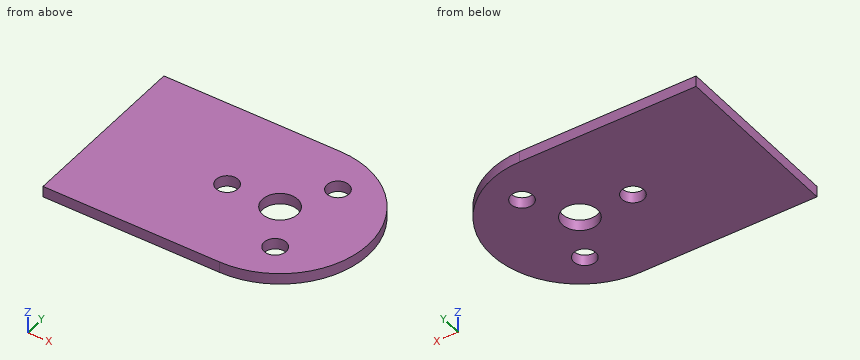
```python
from build123d import *

# Parameters (mm, degrees)
SKETCH1_R           = 5.08
SKETCH1_R_2         = 3.175
BOSS_EXTRUDE1_DEPTH = 3.175


with BuildPart() as part:
    # Sketch1 → Boss-Extrude1 (new body)
    with BuildSketch(Plane.XY):
        with BuildLine():
            Line((22.225, 50.613247917), (-28.575, 50.613247917))
            Line((-28.575, 50.613247917), (-28.575, 101.413247917))
            Line((-28.575, 101.413247917), (22.225, 101.413247917))
            ThreePointArc((22.225, 101.413247917), (47.625, 76.013247917), (22.225, 50.613247917))
        make_face()
        with Locations((22.225, 76.013247917)):
            Circle(SKETCH1_R, mode=Mode.SUBTRACT)
        with Locations((6.985, 76.013247917)):
            Circle(SKETCH1_R_2, mode=Mode.SUBTRACT)
        with Locations((29.845, 89.211475071)):
            Circle(SKETCH1_R_2, mode=Mode.SUBTRACT)
        with Locations((29.845, 62.815020764)):
            Circle(SKETCH1_R_2, mode=Mode.SUBTRACT)
    extrude(amount=BOSS_EXTRUDE1_DEPTH)


solid = part.part
```
Here's how the part is built. I have some questions about the finished solid (model axes, mm). Coordinates: 2 decimals unless noted, no trailing zeros. Write each loop counter-clockwise with the first axis right and the second up, starting at its lowest first coordinate (ties: lowest second). Pieces come first, ordered by that corner, then holes. Notation, with made-up numbers: (15, -15.5) -> (27, -15.5) arc R25 cw to (27, 18.5) -> close; hole circle Ø9 at (-30, 30). An arc over 180 degrees is marked (long way). Use a Markdown table: item, result. Add a question column.
(1) Please list where these lines run through material, in increasing order: line 1 (X direction, y = 75, z = 2.3) (3 decimals); line 2 (X direction, y = 73.5, z = 0.9) (3 decimals); line 3 (X direction, y = 61, z = 2.4) (3 decimals).
(2) If we section it at D-D, the plane y = 68: Write out the boundary of the cut face in (x, z) (3 decimals), and give its area (3 significant figures).
(3) If we section it at B-B, the plane y = 91.5: Write out the boundary of the cut face in (x, z) (3 decimals).
(4) If we section it at A-A, the plane x = 21: Write out the boundary of the cut face in (y, z) (3 decimals), and give its area (3 significant figures).
(5) If we section it at C-C, the plane z = 2.6: Write out the boundary of the cut face in (x, y) (3 decimals).
Outcome:
| question | item | result |
|---|---|---|
| 1 | line 1 | x = -28.575 to 3.976, 9.994 to 17.247, 27.203 to 47.605 |
| 1 | line 2 | x = -28.575 to 5.045, 8.925 to 17.81, 26.64 to 47.5 |
| 1 | line 3 | x = -28.575 to 27.24, 32.45 to 42.713 |
| 2 | outline | (-28.575, 0) -> (46.328, 0) -> (46.328, 3.175) -> (-28.575, 3.175) -> close |
| 2 | area | 238 mm^2 |
| 3 | outline | (-28.575, 0) -> (27.644, 0) -> (27.644, 3.175) -> (-28.575, 3.175) -> close; (32.046, 0) -> (42.358, 0) -> (42.358, 3.175) -> (32.046, 3.175) -> close |
| 4 | outline | (50.613, 0) -> (71.083, 0) -> (71.083, 3.175) -> (50.613, 3.175) -> close; (80.943, 0) -> (101.413, 0) -> (101.413, 3.175) -> (80.943, 3.175) -> close |
| 4 | area | 130 mm^2 |
| 5 | outline | (-28.575, 50.613) -> (22.225, 50.613) arc R25.4 ccw to (22.225, 101.413) -> (-28.575, 101.413) -> close; hole circle Ø6.35 at (6.985, 76.013); hole circle Ø10.16 at (22.225, 76.013); hole circle Ø6.35 at (29.845, 62.815); hole circle Ø6.35 at (29.845, 89.211) |
